Check sheet for the modelled part. Datum: model origin and axes. Units: mm. A direction names the side the tool comes from. Give positions to 0.01 mm unless a question says otherwise; leave off trailing zeros. Order: outer loops, then holes, each group sorted by start corner. A loop starts at its lowest first (then second) coordinate and runs counter-clockwise, first axis right, second up.
from build123d import *

# Parameters (mm, degrees)
F0_W     = 139.7
F0_H     = 76.2
F0_R     = 3.429
F1_DEPTH = 6.35
F2_W     = 6.35
F2_H     = 20.32
F2_H_2   = 76.2
F3_DEPTH = 12.7
F5_DEPTH = 114.301
F6_R     = 3.175
F7_DEPTH = 6.35


# Not quite as in the source:
# - a feature names something its author has since deleted; it is built from what else it names


with BuildPart() as f1:
    # F0 (on Top) → F1 (new body)
    with BuildSketch(Plane.XY):
        Rectangle(F0_W, F0_H)
        Polygon((-63.5, -9.525), (-50.8, -31.75), (-63.5, -31.75), align=None, mode=Mode.SUBTRACT)
        Polygon((-50.8, -25.4), (-63.5, -3.175), (-50.8, -3.175), align=None, mode=Mode.SUBTRACT)
        Polygon((-31.75, -31.75), (-31.75, -3.175), (-6.35, -3.175), align=None, mode=Mode.SUBTRACT)
        with Locations((0, -20.955)):
            Circle(F0_R, mode=Mode.SUBTRACT)
        Polygon((50.8, -31.75), (63.5, -9.525), (63.5, -31.75), align=None, mode=Mode.SUBTRACT)
        Polygon((31.75, -31.75), (6.35, -3.175), (31.75, -3.175), align=None, mode=Mode.SUBTRACT)
        Polygon((63.5, -3.175), (50.8, -25.4), (50.8, -3.175), align=None, mode=Mode.SUBTRACT)
        Polygon((-50.8, 25.4), (-50.8, 3.175), (-63.5, 3.175), align=None, mode=Mode.SUBTRACT)
        Polygon((-6.35, 3.175), (-31.75, 3.175), (-31.75, 31.75), align=None, mode=Mode.SUBTRACT)
        Polygon((-50.8, 31.75), (-63.5, 9.525), (-63.5, 31.75), align=None, mode=Mode.SUBTRACT)
        Polygon((6.35, 3.175), (31.75, 31.75), (31.75, 3.175), align=None, mode=Mode.SUBTRACT)
        Polygon((63.5, 3.175), (50.8, 3.175), (50.8, 25.4), align=None, mode=Mode.SUBTRACT)
        with Locations((0, 20.955)):
            Circle(F0_R, mode=Mode.SUBTRACT)
        Polygon((63.5, 9.525), (50.8, 31.75), (63.5, 31.75), align=None, mode=Mode.SUBTRACT)
    extrude(amount=F1_DEPTH)

    # F2 (on face) → F3 (join)
    with BuildSketch(Plane.XY.offset(6.35)):
        with Locations((41.275, -48.26)):
            Rectangle(F2_W, F2_H)
        with Locations((41.275, 0)):
            Rectangle(F2_W, F2_H_2)
        with Locations((41.275, 48.26)):
            Rectangle(F2_W, F2_H)
        with Locations((-41.275, 48.26)):
            Rectangle(F2_W, F2_H)
        with Locations((-41.275, 0)):
            Rectangle(F2_W, F2_H_2)
        with Locations((-41.275, -48.26)):
            Rectangle(F2_W, F2_H)
    extrude(amount=F3_DEPTH)

    # F4 (on face) → F5 (cut, through all)
    with BuildSketch(Plane.YZ.offset(44.45)):
        Polygon((-48.26, 8.89), (-55.88, 16.51), (-55.88, 8.89), align=None)
        Polygon((-45.72, 16.51), (-53.34, 16.51), (-45.72, 8.89), align=None)
        Polygon((-40.64, 16.51), (-33.02, 8.89), (-33.02, 16.51), align=None)
        Polygon((-43.18, 8.89), (-35.56, 8.89), (-43.18, 16.51), align=None)
        Polygon((-27.94, 16.51), (-20.32, 8.89), (-20.32, 16.51), align=None)
        Polygon((-30.48, 8.89), (-22.86, 8.89), (-30.48, 16.51), align=None)
        Polygon((-15.24, 16.51), (-7.62, 8.89), (-7.62, 16.51), align=None)
        Polygon((-17.78, 8.89), (-10.16, 8.89), (-17.78, 16.51), align=None)
        Polygon((-2.54, 16.51), (5.08, 8.89), (5.08, 16.51), align=None)
        Polygon((-5.08, 8.89), (2.54, 8.89), (-5.08, 16.51), align=None)
        Polygon((10.16, 16.51), (17.78, 8.89), (17.78, 16.51), align=None)
        Polygon((7.62, 8.89), (15.24, 8.89), (7.62, 16.51), align=None)
        Polygon((22.86, 16.51), (30.48, 8.89), (30.48, 16.51), align=None)
        Polygon((20.32, 8.89), (27.94, 8.89), (20.32, 16.51), align=None)
        Polygon((35.56, 16.51), (43.18, 8.89), (43.18, 16.51), align=None)
        Polygon((33.02, 8.89), (40.64, 8.89), (33.02, 16.51), align=None)
        Polygon((48.26, 16.51), (55.88, 8.89), (55.88, 16.51), align=None)
        Polygon((45.72, 8.89), (53.34, 8.89), (45.72, 16.51), align=None)
    extrude(amount=-F5_DEPTH, mode=Mode.SUBTRACT)

    # F6 (on face) → F7 (join)
    with BuildSketch(Plane(origin=(0, 0, 6.35), x_dir=(1, 0, 0), z_dir=(0, 0, -1))):
        with BuildLine():
            ThreePointArc((-44.45, 55.245), (-41.275, 52.07), (-38.1, 55.245))
            ThreePointArc((-38.1, 55.245), (-39.0299359697, 57.4900640303), (-41.275, 58.42))
            ThreePointArc((-41.275, 58.42), (-43.5200640303, 57.4900640303), (-44.45, 55.245))
        make_face()
        with Locations((41.275, 55.245)):
            Circle(F6_R)
        with Locations((-41.275, -55.245)):
            Circle(F6_R)
        with Locations((41.275, -55.245)):
            Circle(F6_R)
    extrude(amount=F7_DEPTH)


solid = f1.part
1) Depth check by flat-ended pin: pin 1 Ø12 at (x, y) = (-53.5, 22.5) entering from +Z; pin 2 Ø2 at (x, y) = (0, -22) entering from +Z; pin 3 Ø6.5 at (y, z) = (16.5, 12.5) entering from +X; pin 4 Ø5 at (x, z) = (18.5, 7.5) entering from +Y. Enter the tip coordinate at first touch or a pass-through.
Recorded:
pin 1: stops at z = 6.35
pin 2: passes through
pin 3: stops at x = 44.45
pin 4: stops at y = 38.1
2) Section check C-C, the plane x = 25. Record the cut outline in (y, z) (3 decimals).
Recorded:
outline: (-38.1, 0) - (-24.156, 0) - (-24.156, 6.35) - (-38.1, 6.35) - close; (-3.175, 0) - (3.175, 0) - (3.175, 6.35) - (-3.175, 6.35) - close; (24.156, 0) - (38.1, 0) - (38.1, 6.35) - (24.156, 6.35) - close
3) Section check B-B, the plane z = 2.75. State how many separate pieces and enclosed holes the cut face has, then the cut area to 3 significant figures.
Recorded:
separate pieces: 5
enclosed holes: 14
area: 8,120 mm2
4) Set-up check for faces 1 (the face through (57.24, 20.48, 3.13)), 2 (the face through (38.935, 53.099, 3.219)), 3 (the face through (44, 58, 6.35)): record each of +Z, -Z, +X, -X, +Y, -Y from which the full face is reachable in a straight line by a thin tool's end or side.
Recorded:
face 1: +Z, -Z
face 2: -Z
face 3: -Z, +X, +Y
5) Draft check along Y on faces 4 (the face through (41.32, 13.92, 12.75)), 5 (the face through (69.85, -1, 3)), 6 (the face through (-57.24, 14.13, 3.13)). Enter one of: +Y half, -Y half, draft (parallel to the pull), parting line (faces both ways), or undercut.
Recorded:
face 4: undercut
face 5: draft
face 6: undercut
6) Material ranges on L1, parallel to Y at x = 0, z = 3.75; L2, parallel to X at y = 18, z = 11; L3, parallel to X at y = -26.5, z = 1.5, recorded low to high.
Recorded:
L1: y = -38.1 to -24.38, -17.53 to 17.53, 24.38 to 38.1
L2: x = -44.45 to -38.1, 38.1 to 44.45
L3: x = -69.85 to -63.5, -53.8 to -31.75, -27.08 to 27.08, 31.75 to 53.8, 63.5 to 69.85
7) Section check A-A, the plane x = 0. Record the cut outline in (y, z), then the cut area to 3 significant figures.
Recorded:
outline: (-38.1, 0) - (-24.38, 0) - (-24.38, 6.35) - (-38.1, 6.35) - close; (-17.53, 0) - (17.53, 0) - (17.53, 6.35) - (-17.53, 6.35) - close; (24.38, 0) - (38.1, 0) - (38.1, 6.35) - (24.38, 6.35) - close
area: 397 mm2
